Design review of the part built by this model. Coordinates are the model's own, in mm. A direction names the side the tool comes from. Round coordinates to 2 decimals unless told otherwise and drop trailing zeros. Loops run counter-clockwise (first coordinate to the right, second up) from the corner with the lowest first, then second, coordinate; pieces in that order, holes last. Notation, with made-up numbers: (35.25, 85.5) - (41.25, 85.5) arc R23 cw to (41.25, 93.5) - close; hole circle Ø2 at (13.25, -40). An arc over 180 degrees is marked (long way). Return JSON: item names as keys, results as strings. Group by question number.
from build123d import *

# Parameters (mm, degrees)
SKETCH1_W                            = 15.24
SKETCH1_H                            = 2.54
BASE_EXTRUDE_DEPTH                   = 1.27
PIN_DEPTH                            = 0.3175
PIN_CHAMFER_SIZE2                    = 0.184896879
PIN_CHAMFER_SIZE                     = 0.508
PIN_PATTERN_COUNT                    = 3
PIN_PATTERN_PITCH                    = 5.08
PIN_CHAMFER_OF_PIN_PATTERN_SIZE2     = 0.184896879
PIN_CHAMFER_OF_PIN_PATTERN_SIZE      = 0.508
PIN_2_DEPTH                          = 0.3175
PIN_2_CHAMFER_SIZE2                  = 0.184896879
PIN_2_CHAMFER_SIZE                   = 0.508
PIN_2_PATTERN_COUNT                  = 3
PIN_2_PATTERN_PITCH                  = 5.08
PIN_2_CHAMFER_OF_PIN_2_PATTERN_SIZE2 = 0.184896879
PIN_2_CHAMFER_OF_PIN_2_PATTERN_SIZE  = 0.508
SV_CUT_DEPTH                         = 4.5
SV_CUT_PATTERN_COUNT                 = 5
SV_CUT_PATTERN_PITCH                 = 2.54
LPATTERN1_COUNT                      = 3
LPATTERN1_PITCH                      = 2.54


with BuildPart() as part:
    # Sketch1 → Base Extrude (new body, symmetric)
    with BuildSketch(Plane(origin=(0, 0, 0), x_dir=(1, 0, 0), z_dir=(0, 1, 0))):
        with Locations((6.35, 0)):
            Rectangle(SKETCH1_W, SKETCH1_H)
    extrude(amount=BASE_EXTRUDE_DEPTH, both=True)

    # Sketch8 → Pin (add, symmetric)
    with BuildSketch(Plane(origin=(0, 0, 0), x_dir=(0, 0, -1), z_dir=(1, 0, 0))):
        with BuildLine():
            Line((0.32004, -1.087), (0.32004, 5.262))
            Line((0.32004, 5.262), (0.135143121, 5.77))
            Line((0.135143121, 5.77), (-0.130063121, 5.77))
            Line((-0.130063121, 5.77), (-0.31496, 5.262))
            Line((-0.31496, 5.262), (-0.31496, -1.214))
            ThreePointArc((-0.31496, -1.214), (-0.01738049, -1.93242049), (0.70104, -2.23))
            Line((0.70104, -2.23), (2.142, -2.23))
            Line((2.142, -2.23), (2.65, -2.045103121))
            Line((2.65, -2.045103121), (2.65, -1.779896879))
            Line((2.65, -1.779896879), (2.142, -1.595))
            Line((2.142, -1.595), (0.82804, -1.595))
            ThreePointArc((0.82804, -1.595), (0.468829755, -1.446210245), (0.32004, -1.087))
        make_face()
    pin = extrude(amount=PIN_DEPTH, both=True)

    # Pin Chamfer
    pin_chamfer_edges = [part.edges().sort_by_distance(p)[0] for p in [
        (0.3175, -1.9125, -2.65),
        (-0.3175, 5.77, -0.00254),
        (-0.3175, -1.9125, -2.65),
        (0.3175, 5.77, -0.00254),
    ]]
    chamfer(pin_chamfer_edges, length=PIN_CHAMFER_SIZE, length2=PIN_CHAMFER_SIZE2)

    # Pin Pattern: Pin ×3
    with Locations(*[(i * PIN_PATTERN_PITCH, 0, 0) for i in range(1, PIN_PATTERN_COUNT)]):
        add(pin)

    # Pin Chamfer of Pin Pattern
    pin_chamfer_of_pin_pattern_edges = [part.edges().sort_by_distance(p)[0] for p in [
        (5.3975, -1.9125, -2.65),
        (4.7625, 5.77, -0.00254),
        (4.7625, -1.9125, -2.65),
        (5.3975, 5.77, -0.00254),
        (10.4775, -1.9125, -2.65),
        (9.8425, 5.77, -0.00254),
        (9.8425, -1.9125, -2.65),
        (10.4775, 5.77, -0.00254),
    ]]
    chamfer(pin_chamfer_of_pin_pattern_edges, length=PIN_CHAMFER_OF_PIN_PATTERN_SIZE, length2=PIN_CHAMFER_OF_PIN_PATTERN_SIZE2)

    # Sketch9 → Pin 2 (add, symmetric)
    with BuildSketch(Plane(origin=(2.54, 0, 0), x_dir=(0, 0, -1), z_dir=(1, 0, 0))):
        with BuildLine():
            Line((-0.32004, -1.087), (-0.32004, 5.262))
            Line((-0.32004, 5.262), (-0.135143121, 5.77))
            Line((-0.135143121, 5.77), (0.130063121, 5.77))
            Line((0.130063121, 5.77), (0.31496, 5.262))
            Line((0.31496, 5.262), (0.31496, -1.214))
            ThreePointArc((0.31496, -1.214), (0.01738049, -1.93242049), (-0.70104, -2.23))
            Line((-0.70104, -2.23), (-2.14454, -2.23))
            Line((-2.14454, -2.23), (-2.65254, -2.045103121))
            Line((-2.65254, -2.045103121), (-2.65254, -1.779896879))
            Line((-2.65254, -1.779896879), (-2.14454, -1.595))
            Line((-2.14454, -1.595), (-0.82804, -1.595))
            ThreePointArc((-0.82804, -1.595), (-0.468829755, -1.446210245), (-0.32004, -1.087))
        make_face()
    pin_2 = extrude(amount=PIN_2_DEPTH, both=True)

    # Pin 2 Chamfer
    pin_2_chamfer_edges = [part.edges().sort_by_distance(p)[0] for p in [
        (2.8575, -1.9125, 2.65254),
        (2.2225, -1.9125, 2.65254),
        (2.2225, 5.77, 0.00254),
        (2.8575, 5.77, 0.00254),
    ]]
    chamfer(pin_2_chamfer_edges, length=PIN_2_CHAMFER_SIZE, length2=PIN_2_CHAMFER_SIZE2)

    # Pin 2 Pattern: Pin 2 ×3
    with Locations(*[(i * PIN_2_PATTERN_PITCH, 0, 0) for i in range(1, PIN_2_PATTERN_COUNT)]):
        add(pin_2)

    # Pin 2 Chamfer of Pin 2 Pattern
    pin_2_chamfer_of_pin_2_pattern_edges = [part.edges().sort_by_distance(p)[0] for p in [
        (7.9375, -1.9125, 2.65254),
        (7.3025, -1.9125, 2.65254),
        (7.3025, 5.77, 0.00254),
        (7.9375, 5.77, 0.00254),
        (13.0175, -1.9125, 2.65254),
        (12.3825, -1.9125, 2.65254),
        (12.3825, 5.77, 0.00254),
        (13.0175, 5.77, 0.00254),
    ]]
    chamfer(pin_2_chamfer_of_pin_2_pattern_edges, length=PIN_2_CHAMFER_OF_PIN_2_PATTERN_SIZE, length2=PIN_2_CHAMFER_OF_PIN_2_PATTERN_SIZE2)

    # Sketch15 → SV Cut (cut, through all)
    with BuildSketch(Plane(origin=(0, 1.27, 0), x_dir=(-1, 0, 0), z_dir=(0, 1, 0))):
        Polygon((-3.556, 1.27), (-3.702646976, 1.016), (-3.917353024, 1.016), (-4.064, 1.27), align=None)
        Polygon((-4.064, -1.27), (-3.917353024, -1.016), (-3.702646976, -1.016), (-3.556, -1.27), align=None)
    sv_cut = extrude(amount=-SV_CUT_DEPTH, mode=Mode.SUBTRACT)

    # SV Cut Pattern: SV Cut ×5
    with Locations(*[(i * SV_CUT_PATTERN_PITCH, 0, 0) for i in range(1, SV_CUT_PATTERN_COUNT)]):
        add(sv_cut, mode=Mode.SUBTRACT)

    # LPattern1: SV Cut ×3
    with Locations(*[(-i * LPATTERN1_PITCH, 0, 0) for i in range(1, LPATTERN1_COUNT)]):
        add(sv_cut, mode=Mode.SUBTRACT)


solid = part.part
Q1. Insertion check: pin 1 Ø0.8 at (y, z) = (-2, -1) entering from -X; pin 2 Ø3 at (x, z) = (3, -1.5) entering from -Y; pin 3 Ø0.6 at (x, y) = (12.5, 0) entering from +Z. Each pin has a flat end and moves straight along its axis. Give the tip position at first contact, or say it passes through.
Q2. Add section D-D, the plane x = 7. State the section outline as (y, z) points, plus the area to 3 significant figures.
Q3. Add section C-C, the plane z = -0.5. State the section outline as (x, y) points, plus the area to 3 significant figures.
Q4. For line 1 (X direction, y = 4, z = 0.2); line 2 (X direction, y = 0, z = -1.1); line 3 (Y direction, x = 3.25, z = 0.7), list the stretches that pass through material, from the lowest coordinate up.
Q5. Add section A-A, the plane z = 1.5. State the section outline as (x, y) points (1 decimal).
Q6. Draft analysis for pull direction X (two halves, no side actions). For faces 1 (the cylindrical face through (2.54, -1.94, -0.01)), 2 (the flat face through (-0.318, -2, -1)), 3 (the cylindrical face through (0, -1.94, 0.01)), state which applies: pulls with the +X half, pulls with the -X half, needs draft (parallel to the pull), parting line crosses it, or undercut.
Q7. Add section B-B, the plane y = 2.75. State the section outline as (x, z) points, plus the area to 3 significant figures.
Q8. Tool access review of faces 4 (the flat face through (5, 0, -1.27)), 5 (the flat face through (3, 0, 1.27)), 6 (the flat face through (10.478, -2, -1)): name each direction out of +Z, -Z, +X, -X, +Y, -Y from which nothing blocks a thin tool from reaching the whole face with its end or side.
Evaluation:
{
 "1": {"pin 1": "x = -0.32", "pin 2": "y = -1.94", "pin 3": "z = 1.27"},
 "2": {"outline": "(-1.27, -1.27) - (1.27, -1.27) - (1.27, 1.27) - (-1.27, 1.27) - close", "area": "6.45 mm²"},
 "3": {"outline": "(-1.27, -1.27) - (13.97, -1.27) - (13.97, 1.27) - (-1.27, 1.27) - close; (-0.32, -2.21) - (0.32, -2.21) - (0.32, -1.47) - (-0.32, -1.47) - close; (4.76, -2.21) - (5.4, -2.21) - (5.4, -1.47) - (4.76, -1.47) - close; (9.84, -2.21) - (10.48, -2.21) - (10.48, -1.47) - (9.84, -1.47) - close", "area": "40.1 mm²"},
 "4": {"line 1": "-0.32 to 0.32, 2.22 to 2.86, 4.76 to 5.4, 7.3 to 7.94, 9.84 to 10.48, 12.38 to 13.02", "line 2": "-1.11 to 1.11, 1.43 to 3.65, 3.97 to 6.19, 6.51 to 8.73, 9.05 to 11.27, 11.59 to 13.81", "line 3": "-1.27 to 1.27"},
 "5": {"outline": "(2.2, -2.2) - (2.9, -2.2) - (2.9, -1.6) - (2.2, -1.6) - close; (7.3, -2.2) - (7.9, -2.2) - (7.9, -1.6) - (7.3, -1.6) - close; (12.4, -2.2) - (13, -2.2) - (13, -1.6) - (12.4, -1.6) - close"},
 "6": {"face 1": "undercut", "face 2": "pulls with the -X half", "face 3": "needs draft"},
 "7": {"outline": "(-0.32, -0.32) - (0.32, -0.32) - (0.32, 0.31) - (-0.32, 0.31) - close; (2.22, -0.31) - (2.86, -0.31) - (2.86, 0.32) - (2.22, 0.32) - close; (4.76, -0.32) - (5.4, -0.32) - (5.4, 0.31) - (4.76, 0.31) - close; (7.3, -0.31) - (7.94, -0.31) - (7.94, 0.32) - (7.3, 0.32) - close; (9.84, -0.32) - (10.48, -0.32) - (10.48, 0.31) - (9.84, 0.31) - close; (12.38, -0.31) - (13.02, -0.31) - (13.02, 0.32) - (12.38, 0.32) - close", "area": "2.42 mm²"},
 "8": {"face 4": "-Z, +X, -X, +Y", "face 5": "+Z, +X, -X, +Y", "face 6": "+Z, -Z, -Y"}
}
